from build123d import *

# Parameters (mm, degrees)
F0_R     = 10
F0_R_2   = 5
F1_DEPTH = 10
F3_DEPTH = 25
F7_D     = 5
F7_DEPTH = 10.0010001


# Not quite as in the source:
# - a fillet or chamfer that OpenCascade refuses, or shapes differently, is made with other operations: its cross-section is extruded or revolved along the edge and cut away or added


with BuildPart() as f1:
    # F0 (on Top) → F1 (new body, symmetric)
    with BuildSketch(Plane.XY):
        Circle(F0_R)
        Circle(F0_R_2, mode=Mode.SUBTRACT)
    extrude(amount=F1_DEPTH, both=True)

    # F2 (on face) → F3 (cut)
    with BuildSketch(Plane.XY.offset(10)):
        with BuildLine():
            Line((2.5, -4.3301270189), (2.5, 4.3301270189))
            ThreePointArc((2.5, 4.3301270189), (0, 5), (-2.5, 4.3301270189))
            Line((-2.5, 4.3301270189), (-2.5, -4.3301270189))
            ThreePointArc((-2.5, -4.3301270189), (0, -5), (2.5, -4.3301270189))
        make_face()
        with BuildLine():
            Line((2.5, 4.3301270189), (2.5, 7.5))
            Line((2.5, 7.5), (-2.5, 7.5))
            Line((-2.5, 7.5), (-2.5, 4.3301270189))
            ThreePointArc((-2.5, 4.3301270189), (0, 5), (2.5, 4.3301270189))
        make_face()
        with BuildLine():
            Line((2.5, -7.5), (2.5, -4.3301270189))
            ThreePointArc((2.5, -4.3301270189), (0, -5), (-2.5, -4.3301270189))
            Line((-2.5, -4.3301270189), (-2.5, -7.5))
            Line((-2.5, -7.5), (2.5, -7.5))
        make_face()
    extrude(amount=-F3_DEPTH, mode=Mode.SUBTRACT)

    # F4: fillet of radius 5 on 1 edges, made by hand

    # F4_s1 → F4_t2 (revolve, cut)
    with BuildSketch(Plane.XZ):
        with BuildLine():
            ThreePointArc((10, 5), (8.5355339059, 8.5355339059), (5, 10))
            Line((5, 10), (10, 10))
            Line((10, 10), (10, 5))
        make_face()
    revolve(axis=Axis((0, 0, 10), (0, 0, 1)), mode=Mode.SUBTRACT)

    # F5: chamfer of 5 on 1 edges, made by hand

    # F5_s1 → F5_t2 (revolve, cut)
    with BuildSketch(Plane.XZ):
        Polygon((10, -5), (5, -10), (10, -10), align=None)
    revolve(axis=Axis((0, 0, -10), (0, 0, 1)), mode=Mode.SUBTRACT)

    # F7 (through all, one way)
    with BuildSketch(Plane.XZ):
        with Locations((0, 0)):
            Circle(F7_D / 2)
    extrude(amount=-F7_DEPTH, mode=Mode.SUBTRACT)


solid = f1.part
Read the model definition and answer for the solid it produces. Units are mm, in the model's axes. A direction names the side the tool comes from. Give positions to 0.01 mm unless a question says otherwise; leave off trailing zeros. Answer as CSV lines item,"result".
Item 1: Each of these flat-tipped pins is pushed along its axis until it touches: pin 1 (5 mm diameter, centred on x = 7, z = -4.5, fed in from +Y); pin 2 (1 mm diameter, centred on x = 5.5, z = 4, fed in from +Y); pin 3 (6 mm diameter, centred on x = 5, z = -2, fed in from +Y). Where does it stop, or does it pass through?
Returned:
pin 1,"stops at y = 8.93"
pin 2,"stops at y = 8.66"
pin 3,"stops at y = 9.8"
Item 2: Consider line 1 (Y direction, x = 0.25, z = 4.5); line 2 (Y direction, x = -4.25, z = 6.5); line 3 (Y direction, x = 6.25, z = 6.5). Determine where each line is inside the solid, lowest interval first. Write a range as [from, to].
Returned:
line 1,"y = [-10, -7.5], [7.5, 10]"
line 2,"y = [-8.8, -2.63], [2.63, 8.8]"
line 3,"y = [-7.51, 7.51]"
Item 3: For faces 3 (the face through (2.385, 8.737, 0.751)), 4 (the face through (5, 0, 0)), 5 (the face through (5, 1.57, -9.76)), determine the directions among +Z, -Z, +X, -X, +Y, -Y from which every point of the face is accessible in a straight line to the end or side of a thin tool.
Returned:
face 3,"+Y"
face 4,"+Z, -Z"
face 5,"-Z"
Item 4: Find section A-A on x = 0. State how many separate pieces and enclosed holes the cut face has, plus the area to 3 significant figures.
Returned:
separate pieces,"3"
enclosed holes,"0"
area,"59.1 mm²"
Item 5: Determine the mould class of faces 1 (the face through (0, 7.5, -5)), 2 (the face through (-2.17, -9.76, 0.07)) for opening direction X: +X half, -X half, draft (parallel to the pull), parting line (faces both ways), or undercut.
Returned:
face 1,"undercut"
face 2,"parting line"
